Geometry check sheet. Reference: the model listing, model coordinates, mm. A direction names the side the tool comes from. Coordinates: 2 decimals unless noted, no trailing zeros. Write each loop counter-clockwise with the first axis right and the second up, starting at its lowest first coordinate (ties: lowest second). Pieces come first, ordered by that corner, then holes.
from build123d import *

# Parameters (mm, degrees)
F0_W     = 51.2064
F0_H     = 85.09
F1_DEPTH = 6.604
F2_R     = 3.175
F3_DEPTH = 95.21702
F4_W     = 51.2064
F4_H     = 44.45
F5_DEPTH = 5.95932
F6_R     = 5.08
F7_W     = 5.334
F7_H     = 43.18
F8_DEPTH = 25.4


with BuildPart() as f1:
    # F0 (on Top) → F1 (new body)
    with BuildSketch(Plane.XY):
        with Locations((-4.726471, -15.027478)):
            Rectangle(F0_W, F0_H)
    extrude(amount=-F1_DEPTH)

    # F2 (on face) → F3 (cut)
    with BuildSketch(Plane.YZ.offset(20.876729)):
        with Locations((18.137634, -3.302)):
            Circle(F2_R)
        with Locations((-47.881499, -3.302)):
            Circle(F2_R)
    extrude(amount=-F3_DEPTH, mode=Mode.SUBTRACT)

    # F4 (on face) → F5 (cut)
    with BuildSketch(Plane(origin=(0, 0, -6.604), x_dir=(1, 0, 0), z_dir=(0, 0, -1))):
        with Locations((-4.726471, 15.027478)):
            Rectangle(F4_W, F4_H)
    extrude(amount=-F5_DEPTH, mode=Mode.SUBTRACT)

    # F6
    f6_edges = [f1.edges().sort_by_distance(p)[0] for p in [
        (-4.726471, -37.252478, -6.604),
        (-4.726471, -57.572478, -6.604),
        (-4.726471, 7.197522, -6.604),
        (-4.726471, 27.517522, -6.604),
    ]]
    fillet(f6_edges, radius=F6_R)

    # F7 (on face) → F8 (cut)
    with BuildSketch(Plane.XY):
        with Locations((-27.662671, -14.693605)):
            Rectangle(F7_W, F7_H)
        with Locations((18.209729, -14.693605)):
            Rectangle(F7_W, F7_H)
    extrude(amount=-F8_DEPTH, mode=Mode.SUBTRACT)


solid = f1.part
1. Sectioned sample at A-A, the plane z = -4.5. Record the boundary of the cut face in (x, y), and give its area (3 significant figures).
Computed values:
outline: (-30.33, -56.61) - (20.88, -56.61) - (20.88, -50.82) - (-30.33, -50.82) - close; (-30.33, -44.94) - (20.88, -44.94) - (20.88, -38.22) - (-30.33, -38.22) - close; (-30.33, 8.16) - (20.88, 8.16) - (20.88, 15.2) - (-30.33, 15.2) - close; (-30.33, 21.08) - (20.88, 21.08) - (20.88, 26.55) - (-30.33, 26.55) - close
area: 1,280 mm2
2. Sectioned sample at C-C, the plane y = -47. Record the boundary of the cut face in (x, z), and give its area (3 significant figures).
Computed values:
outline: (-30.33, -6.6) - (20.88, -6.6) - (20.88, -6.35) - (-30.33, -6.35) - close; (-30.33, -0.25) - (20.88, -0.25) - (20.88, 0) - (-30.33, 0) - close
area: 25.8 mm2
3. Sectioned sample at B-B, the plane x = 17.5. Give the number of separate pieces and of enclosed holes in the cut face, and give its area (3 significant figures).
Computed values:
separate pieces: 2
enclosed holes: 2
area: 184 mm2
4. Thickness scan on line 1 along Y through (x, z) = (-15, -1.75); line 2 along Y through (x, z) = (-25.5, -4.75); line 3 along Y through (x, z) = (10.5, -0.5). Record the ranges inside material, lowest first.
Computed values:
line 1: y = -57.57 to -50.65, -45.11 to -37.26, 7.2 to 15.37, 20.91 to 27.51
line 2: y = -56.42 to -50.71, -45.06 to -38.41, 8.35 to 15.31, 20.96 to 26.36
line 3: y = -57.57 to -49.37, -46.39 to 16.64, 19.63 to 27.52
5. Access from +Z, -Z, +X, -X, +Y, -Y to the whole of each face (thin tool, end or side, straight path). Record for faces 1 (the flat face through (-5, -15, -0.645)), 2 (the cylindrical face through (-4.368, 26.069, -5.076)).
Computed values:
face 1: -Z, +X, -X
face 2: -Z, +X, -X, +Y
6. Gauge pin test, flat ends, axial feed: pin 1 Ø8 at (x, y) = (-22.5, 2.5) entering from +Z; pin 2 Ø0.7 at (y, z) = (-11, -0.5) entering from +X; pin 3 Ø12 at (x, y) = (-3, -27) entering from -Z. Record the tip position at first contact, or that the pin passes through.
Computed values:
pin 1: stops at z = 0
pin 2: stops at x = 15.54
pin 3: stops at z = -0.64
7. Draft check along Z on faces 3 (the cylindrical face through (-4.368, -51.053, -3.162)), 4 (the flat face through (-30.33, -44.7, -1.8)), 5 (the cylindrical face through (-4.37, 8.73, -5.16)), 6 (the cylindrical face through (-4.368, 14.966, -3.162)). Enter one of: released by +Z, released by -Z, zero draft, split by the parting line, or undercut.
Computed values:
face 3: undercut
face 4: zero draft
face 5: released by -Z
face 6: undercut
